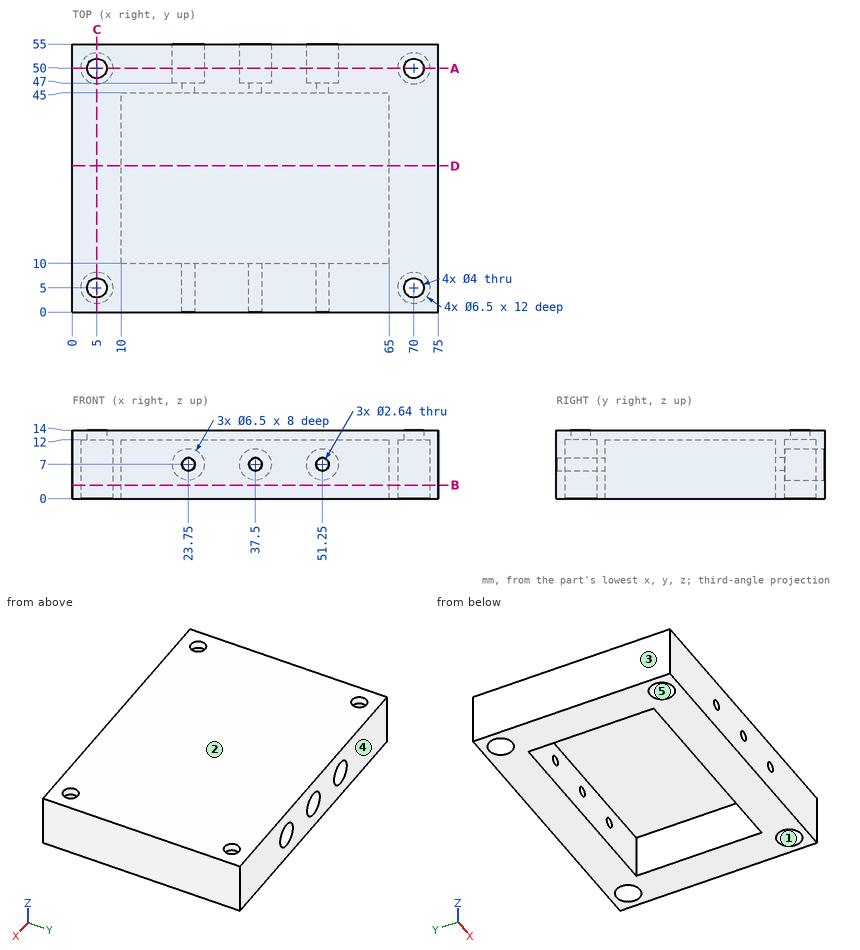
Can you work these out from the drawing? Everything is in mm from the part's minimum corner. A direction names the side the tool comes from. Coordinates: 2 decimals unless noted, no trailing zeros. Loops run counter-clockwise (first coordinate to the right, second up) from the corner with the lowest first, then second, coordinate; pieces in that order, holes last.
1. Imagine slicing it at B-B, the plane z = 2.75. Please give me the cut outline in (x, y).
2. I need wall thicknesses on L1, parallel to X at y = 37.5, z = 3.25; L2, parallel to Y at x = 40.5, z = 2.25; L3, parallel to X at y = 49.5, z = 7. Which ranges of each line are inside material? Lowest first, please.
3. For the marked faces 1 and 2, which set-ups out of +Z, -Z, +X, -X, +Y, -Y let a thin tool reach every point of the face, with its end or its side?
4. Imagine slicing it at D-D, the plane y = 30. Please give me the cut outline in (x, z), and give its area (3 significant figures).
5. For P1, Ø1.6, axis at x = 23.75, z = 7, coming from the +Y side; P2, Ø3, axis at x = 14.5, y = 17, coming from the -Z side; P3, Ø4, axis at x = 51.25, z = 7, coming from the +Y side, each with a flat end and sliding along its axis, tell me the tip position at first contact or that it passes through.
6. If we mould it in two halves opening along X, with no side actions, what happens to the marked faces 3, 4 and 5? For each: pulls with the +X half, pulls with the -X half, needs draft (parallel to the pull), parting line crosses it, or undercut.
7. Imagine slicing it at A-A, the plane y = 50. Please give me the cut outline in (x, z), and give its area (3 significant figures).
8. Imagine slicing it at C-C, the plane x = 5. Please give me the cut outline in (y, z), and give its area (3 significant figures).
Taken from the geometry:
1. outline: (0, 0) - (75, 0) - (75, 55) - (0, 55) - close; hole circle Ø6.5 at (5, 5); hole circle Ø6.5 at (5, 50); hole (10, 10) - (65, 10) - (65, 45) - (10, 45) - close; hole circle Ø6.5 at (70, 5); hole circle Ø6.5 at (70, 50)
2. L1: x = 0 to 10, 65 to 75
2. L2: y = 0 to 10, 45 to 55
2. L3: x = 0 to 1.79, 8.21 to 20.5, 27 to 34.25, 40.75 to 48, 54.5 to 66.79, 73.21 to 75
3. face 1: -Z
3. face 2: +Z, +X, -X, +Y, -Y
4. outline: (0, 0) - (10, 0) - (10, 12) - (65, 12) - (65, 0) - (75, 0) - (75, 14) - (0, 14) - close
4. area: 390 mm2
5. P1: passes through
5. P2: stops at z = 12
5. P3: stops at y = 47
6. face 3: pulls with the -X half
6. face 4: needs draft
6. face 5: undercut
7. outline: (0, 0) - (1.75, 0) - (1.75, 12) - (3, 12) - (3, 14) - (0, 14) - close; (7, 12) - (8.25, 12) - (8.25, 0) - (66.75, 0) - (66.75, 12) - (68, 12) - (68, 14) - (7, 14) - close; (72, 12) - (73.25, 12) - (73.25, 0) - (75, 0) - (75, 14) - (72, 14) - close; hole circle Ø6.5 at (23.75, 7); hole circle Ø6.5 at (37.5, 7); hole circle Ø6.5 at (51.25, 7)
7. area: 778 mm2
8. outline: (0, 0) - (1.75, 0) - (1.75, 12) - (3, 12) - (3, 14) - (0, 14) - close; (7, 12) - (8.25, 12) - (8.25, 0) - (46.75, 0) - (46.75, 12) - (48, 12) - (48, 14) - (7, 14) - close; (52, 12) - (53.25, 12) - (53.25, 0) - (55, 0) - (55, 14) - (52, 14) - close
8. area: 598 mm2
